Autodesk Inventor part; units mm, degrees
ref_plane "YZ Plane" through (0, 0, 0) normal (1, 0, 0) x (0, 1, 0)
ref_plane "XZ Plane" through (0, 0, 0) normal (0, 1, 0) x (-1, 0, 0)
ref_plane "XY Plane" through (0, 0, 0) normal (0, 0, 1) x (1, 0, 0)
sketch "Skizze1" plane through (0, 0, 0) normal (0, 1, 0) x (-1, 0, 0)
  circle A0 centre (0, 0) radius 100
  dimension "d0" = 200
extrude "Extrusion1" add sketch "Skizze1" along normal blind 10
sketch "Skizze2" plane through (0, 10, 0) normal (0, 1, 0) x (1, 0, 0)
  circle A0 centre (0, 0) radius 100
  circle A1 centre (-87, 0) radius 3.1
  dimension "d3" = 6.2
  dimension "d4" = 87
  dimension "d5" = 200
extrude "Extrusion2" cut sketch "Skizze2" against normal through all contours A1
chamfer "Fasen1" distance 4 angle 45 1 edges at (-90.1, 0, 0)
sketch "Skizze3" plane through (0, 10, 0) normal (0, 1, 0) x (1, 0, 0)
  circle A0 centre (-87, 0) radius 3.1
  circle A1 centre (0, 0) radius 100
  line L0 (-97, -24.3105) -> (-97, 24.3105)
  circle A2 centre (0, 0) radius 100
  point P0 (-97, -24.3105)
  dimension "d11" = 10
extrude "Extrusion3" cut sketch "Skizze3" against normal through all contours L0 A1 picked at (-97.7491, 4.0825)
pattern_circular "Runde Anordnung3" count 4 over 360 about axis through (0, -10, 0) along (0, 1, 0) of "Extrusion2", "Fasen1"
pattern_circular "Runde Anordnung4" count 4 over 360 about axis through (0, -10, 0) along (0, 1, 0) of "Extrusion3"
properties part number "plate_lower"
Build history of the part. All positions in model axes, mm. Give positions to 0.01 mm unless a question says otherwise; leave off trailing zeros. Order: outer loops, then holes, each group sorted by start corner. A loop starts at its lowest first (then second) coordinate and runs counter-clockwise, first axis right, second up. Notation, with made-up numbers: M 19,25 L 67,25 A23 cw 67,63 Z; hole C 71,64.25 d10. An arc over 180 degrees is marked long. Use one line per item in the form item = value.
1) Saw through at D-D (x = 87). Give the cut face in (y, z).
Calculated:
outline = M 0,-49.31 L 10,-49.31 L 10,-3.1 L 4,-3.1 L 0,-7.1 Z; M 0,7.1 L 4,3.1 L 10,3.1 L 10,49.31 L 0,49.31 Z
2) Saw through at A-A (x = 0). Give the cut face in (y, z), plus the area to 3 significant figures.
Calculated:
outline = M 0,-97 L 10,-97 L 10,-90.1 L 4,-90.1 L 0,-94.1 Z; M 0,-79.9 L 4,-83.9 L 10,-83.9 L 10,83.9 L 4,83.9 L 0,79.9 Z; M 0,94.1 L 4,90.1 L 10,90.1 L 10,97 L 0,97 Z
area = 1,780 mm2
3) Probe probe 1 along X at (y, z) = (0.75, 4); probe 2 along Z at (x, y) = (-83, 0.5); probe 3 along Z at (x, y) = (-87, 5.2). List the from-to ranges inside material, lowest first.
Calculated:
probe_1 = -97 to -91.93, -82.07 to 82.07, 91.93 to 97
probe_2 = -55.78 to -5.25, 5.25 to 55.78
probe_3 = -49.31 to -3.1, 3.1 to 49.31
4) Saw through at B-B (z = 0). Give the cut face in (x, y), plus the area to 3 significant figures.
Calculated:
outline = M -97,0 L -94.1,0 L -90.1,4 L -90.1,10 L -97,10 Z; M -83.9,4 L -79.9,0 L 79.9,0 L 83.9,4 L 83.9,10 L -83.9,10 Z; M 90.1,4 L 94.1,0 L 97,0 L 97,10 L 90.1,10 Z
area = 1,780 mm2
5) Saw through at C-C (y = 7.25). Give the cut face in (x, z).
Calculated:
outline = M -97,-24.31 A100 ccw -24.31,-97 L 24.31,-97 A100 ccw 97,-24.31 L 97,24.31 A100 ccw 24.31,97 L -24.31,97 A100 ccw -97,24.31 Z; hole C -87,0 d6.2; hole C 0,-87 d6.2; hole C 0,87 d6.2; hole C 87,0 d6.2
6) Two-plate mould, pull along Z, no slides. Class faces 1 (the face through (97, 5, 0)), 2 (the face through (-71.243, 4.93, -70.174)), 3 (the face through (0.931, 7.042, -84.043)), 4 (the face through (-84.043, 7.042, -0.931)): released by +Z, released by -Z, zero draft, split by the parting line, or undercut.
Calculated:
face_1 = zero draft
face_2 = released by -Z
face_3 = undercut
face_4 = undercut
7) Drop flat-ended pins along their axis: pin 1 (4 mm diameter, centred on y = 5, z = -72, fed in from +X); pin 2 (2 mm diameter, centred on y = 3, z = 32, fed in from +X); pin 3 (7 mm diameter, centred on x = 0, z = -87, fed in from -Y). Give the stop position or say it passes through.
Calculated:
pin_1 = 71.41
pin_2 = 95.07
pin_3 = 3.6
